```python
from build123d import *

# Parameters (mm, degrees)
F0_R     = 50
F0_R_2   = 46
F0_R_3   = 43.6
F1_DEPTH = 2
F2_DEPTH = 30
F3_SIZE  = 4


with BuildPart() as f1:
    # F0 (on Top) → F1 (new body)
    with BuildSketch(Plane.XY):
        Circle(F0_R)
        Circle(F0_R_2, mode=Mode.SUBTRACT)
        Circle(F0_R_2)
        Circle(F0_R_3, mode=Mode.SUBTRACT)
        Circle(F0_R_3)
    extrude(amount=F1_DEPTH)

    # F0 (on Top) → F2 (join)
    with BuildSketch(Plane.XY):
        Circle(F0_R_2)
        Circle(F0_R_3, mode=Mode.SUBTRACT)
    extrude(amount=F2_DEPTH)

    # F3
    f3_edges = [f1.edges().sort_by_distance(p)[0] for p in [
        (-43.6, 0, 2),
    ]]
    chamfer(f3_edges, length=F3_SIZE)


solid = f1.part
```
Check sheet for the modelled part. Datum: model origin and axes. Units: mm. A direction names the side the tool comes from. Coordinates: 2 decimals unless noted, no trailing zeros. Write each loop counter-clockwise with the first axis right and the second up, starting at its lowest first coordinate (ties: lowest second). Pieces come first, ordered by that corner, then holes. Notation, with made-up numbers: M 37.25,-3.75 L 81.25,-3.75 A26 ccw 81.25,28.25 Z; hole C -12,-31.5 d1. An arc over 180 degrees is marked long. Write item = value, one per line. Start each with the question number.
1. Mould release check, pull along Y, two halves, no side actions. Record for faces 1 (the conical face through (-8.627, 38.848, 2.194)), 2 (the cylindrical face through (41.587, 13.096, 17.832)), 3 (the flat face through (-1, 1, 0)), 4 (the cylindrical face through (47.69, 15.02, 0.99)): pulls with the +Y half, pulls with the -Y half, needs draft (parallel to the pull), parting line crosses it, or undercut.
2. Thickness scan on probe 1 along X at (y, z) = (0, 18.5); probe 2 along X at (y, z) = (-2, 11). Record the ranges inside material, lowest first.
3. Tool access check on faces 5 (the flat face through (17, -41, 30)), 6 (the cylindrical face through (-5.99, 45.61, 15.8)). Record the directions out of +Z, -Z, +X, -X, +Y, -Y that give a thin tool (end or side, any length) a straight path to the whole face; none if there is none.
4. Sectioned sample at A-A (y = 0). Record the cut outline in (x, z).
5. Go/stop test with flat-tipped pins: pin 1 (3 mm diameter, centred on x = -20, y = 31, fed in from -Z); pin 2 (10 mm diameter, centred on x = 26.5, z = 6.5, fed in from +Y); pin 3 (3 mm diameter, centred on y = -27, z = 24, fed in from +X); pin 4 (3 mm diameter, centred on x = -14.5, z = 5, fed in from -Y). Record where each tip stops, or that it passes through.
6. Sectioned sample at B-B (z = 26). Record the cut outline in (x, y), then the cut area to 3 significant figures.
The answers:
q1.face_1 = undercut
q1.face_2 = undercut
q1.face_3 = needs draft
q1.face_4 = parting line crosses it
q2.probe_1 = -46 to -43.6, 43.6 to 46
q2.probe_2 = -45.96 to -43.55, 43.55 to 45.96
q3.face_5 = +Z, +X, -X, +Y, -Y
q3.face_6 = +Z
q4.outline = M -50,0 L 50,0 L 50,2 L 46,2 L 46,30 L 43.6,30 L 43.6,6 L 39.6,2 L -39.6,2 L -43.6,6 L -43.6,30 L -46,30 L -46,2 L -50,2 Z
q5.pin_1 = 0
q5.pin_2 = 43.69
q5.pin_3 = 38.29
q5.pin_4 = -44.12
q6.outline = C 0,0 d92; hole C 0,0 d87.2
q6.area = 676 mm²
